Here's the drawing with two shaded views (mm, measured from the low corner). I have some questions. Coordinates: 2 decimals unless noted, no trailing zeros. Loops run counter-clockwise (first coordinate to the right, second up) from the corner with the lowest first, then second, coordinate; pieces in that order, holes last. Notation, with made-up numbers: (39, 17.25) - (94, 17.25) arc R37 cw to (94, 56.25) - close; hole circle Ø11 at (74, 58.25). An arc over 180 degrees is marked (long way). One line per item, written item: value. Start each with the question number.
(1) I'm going to push flat-ended pins straight in: P1, Ø1, axis at y = 3, z = 54.5, coming from the +X side; P2, Ø12, axis at y = 2.5, z = 39.5, coming from the -X side; P3, Ø1.5, axis at x = 35.5, y = 14, coming from the -Z side; P4, Ø8, axis at y = 14, z = 60, coming from the -X side (1 decimal). Where does each tip first touch, or does it pass through?
(2) If I drill on line 1 along Y through (x, z) = (49, 69); line 2 along Z through (x, y) = (58.5, 9.75) (1 decimal); line 3 along X through (y, z) = (13.5, 28.5), over which ranges is the centre line in solid material (lowest first)? Write a range as from..to.
(3) If we section it at B-B on y = 16.5: Write out the boundary of the cut face in (x, z).
(4) If we section it at D-D on x = 14: Write out the boundary of the cut face in (y, z), then the cut area to 3 significant figures.
(5) If we section it at C-C on z = 36: Write out the boundary of the cut face in (x, y).
(6) If we mould it in two halves opening along X, with no side actions, what happens to the marked faces 1, 2 and 3? For each: pulls with the +X half, pulls with the -X half, needs draft (parallel to the pull), parting line crosses it, or undercut.
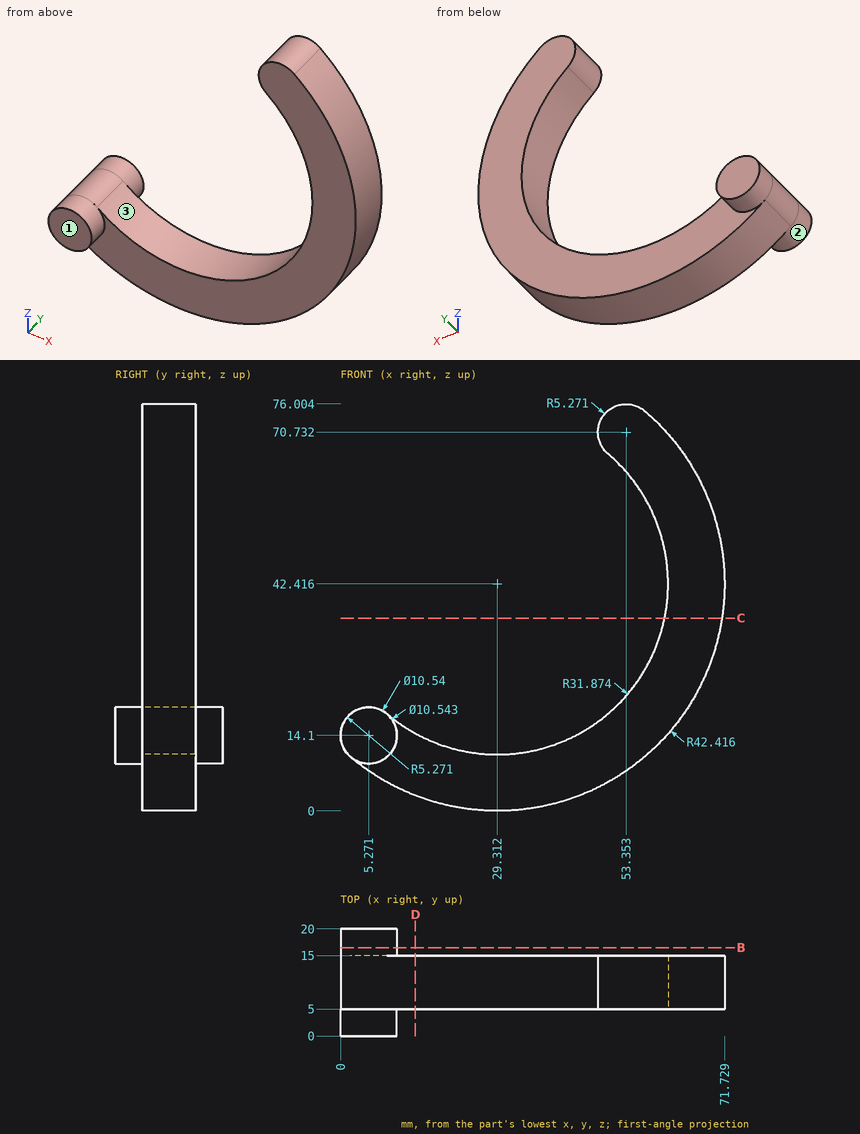
Values:
1. P1: passes through
1. P2: stops at x = 60.07
1. P3: stops at z = 0.35
1. P4: stops at x = 52.8
2. line 1: y = 5..15
2. line 2: z = 11.6..29.6, 55.2..73.2
2. line 3: x = 57.99..69.38
3. outline: circle Ø10.54 at (5.27, 14.1)
4. outline: (5, 2.86) - (15, 2.86) - (15, 14.46) - (5, 14.46) - close
4. area: 116 mm2
5. outline: (60.53, 5) - (71.24, 5) - (71.24, 15) - (60.53, 15) - close
6. face 1: needs draft
6. face 2: parting line crosses it
6. face 3: undercut
